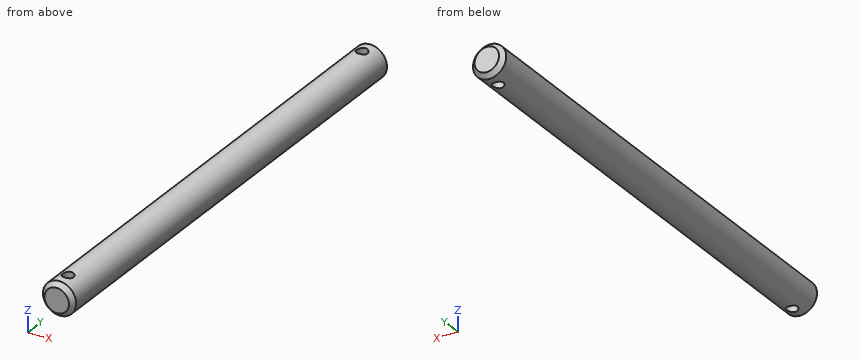
from build123d import *

# Parameters (mm, degrees)
F0_R     = 7.5
F1_DEPTH = 225
F3_R     = 2.5
F4_DEPTH = 15.001
F5_SIZE  = 2
F6_SIZE  = 2


with BuildPart() as f1:
    # F0 (on Front) → F1 (new body)
    with BuildSketch(Plane.XZ):
        Circle(F0_R)
    extrude(amount=F1_DEPTH)

    # F3 (on offset) → F4 (cut, through all)
    with BuildSketch(Plane.XY.offset(7.5)):
        with Locations((0, -8)):
            Circle(F3_R)
        with Locations((0, -217)):
            Circle(F3_R)
    extrude(amount=-F4_DEPTH, mode=Mode.SUBTRACT)

    # F5
    f5_edges = [f1.edges().sort_by_distance(p)[0] for p in [
        (-7.5, -225, 0),
    ]]
    chamfer(f5_edges, length=F5_SIZE)

    # F6
    f6_edges = [f1.edges().sort_by_distance(p)[0] for p in [
        (-7.5, 0, 0),
    ]]
    chamfer(f6_edges, length=F6_SIZE)


solid = f1.part
Geometry: final body of the model. Coordinates: model frame, mm. Coordinates: 2 decimals unless noted, no trailing zeros. Write each loop counter-clockwise with the first axis right and the second up, starting at its lowest first coordinate (ties: lowest second). Pieces come first, ordered by that corner, then holes. Notation, with made-up numbers: (40, 69.25) - (58, 69.25) arc R26 ccw to (58, 105.25) - close; hole circle Ø9 at (43, -37). An arc over 180 degrees is marked (long way). Return JSON: item names as keys, results as strings.
Item 1: Pin query (flat end, axial travel): pin 1 Ø2 at (y, z) = (-160.5, -3) entering from +X; pin 2 Ø4 at (y, z) = (-107.5, 4.5) entering from -X. Return the tip coordinate at first contact, or that it passes through.
Completed:
{"pin 1": "stops at x = 7.23", "pin 2": "stops at x = -7.07"}
Item 2: Section query B-B (y = -8). Output: boundary loops of the cut face in (x, z), and give its area (3 significant figures).
Completed:
{"outline": "(-2.5, -7.07) - (-2.5, 7.07) arc R7.5 ccw to start; (2.5, -7.07) arc R7.5 ccw to (2.5, 7.07) - close", "area": "103 mm2"}
Item 3: Section query A-A (x = 0). Output: boundary loops of the cut face in (y, z).
Completed:
{"outline": "(-225, -5.5) - (-223, -7.5) - (-219.5, -7.5) - (-219.5, 7.5) - (-223, 7.5) - (-225, 5.5) - close; (-214.5, -7.5) - (-10.5, -7.5) - (-10.5, 7.5) - (-214.5, 7.5) - close; (-5.5, -7.5) - (-2, -7.5) - (0, -5.5) - (0, 5.5) - (-2, 7.5) - (-5.5, 7.5) - close"}
Item 4: Line query: L1, parallel to Y at x = 0, z = -0.25; L2, parallel to Y at x = 2.25, z = -5.75; L3, parallel to X at y = -217, z = 4. Output: solid intervals per line, ascending.
Completed:
{"L1": "y = -225 to -219.5, -214.5 to -10.5, -5.5 to 0", "L2": "y = -224.33 to -218.09, -215.91 to -9.09, -6.91 to -0.67", "L3": "x = -6.34 to -2.5, 2.5 to 6.34"}
Item 5: Section query C-C (y = -35). Output: boundary loops of the cut face in (x, z), and give its area (3 significant figures).
Completed:
{"outline": "circle Ø15 at (0, 0)", "area": "177 mm2"}
